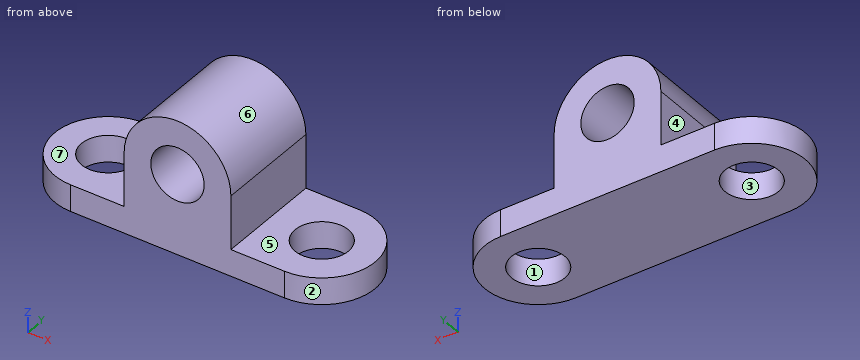
Autodesk Fusion 360 part; units mm, degrees
sketch "Sketch1" plane through (0, 0, 0) normal (0, 0, 1) x (1, 0, 0)
  line L0 (40, -20) -> (-40, -20)
  line L1 (-40, 20) -> (40, 20)
  circle A0 centre (40, 0) radius 10
  circle A1 centre (-40, 0) radius 10
  arc A2 (40, -20) -> (40, 20) centre (40, 0) ccw
  arc A3 (-40, 20) -> (-40, -20) centre (-40, 0) ccw
  dimension "d1" = 80
  dimension "d2" = 40
extrude "Extrude1" add sketch "Sketch1" along normal blind 10
sketch "Sketch2" plane through (0, 0, 0) normal (0, 1, 0) x (1, 0, 0)
  line L0 (-20, -0.1094) -> (20, -0.1094)
  line L1 (20, -0.1094) -> (20, -30.1094)
  line L2 (-20, -30.1094) -> (-20, -0.1094)
  line L3 (-40, 0) -> (-40, -10)
  circle A0 centre (0, -30.1094) radius 20
  circle A1 centre (0, -30.1094) radius 10
  dimension "d9" = 40
  dimension "d10" = 30
  dimension "d11" = 20
  dimension "d12" = 40
  dimension "d13" = 20
extrude "Extrude2" add sketch "Sketch2" along normal mid plane 40
Check sheet for the modelled part. Datum: model origin and axes. Units: mm. Face numbers are marked on the shaded views. A direction names the side the tool comes from. Give positions to 0.01 mm unless a question says otherwise; leave off trailing zeros. Order: outer loops, then holes, each group sorted by start corner. A loop starts at its lowest first (then second) coordinate and runs counter-clockwise, first axis right, second up. Notation, with made-up numbers: M 21.25,6.5 L 55.25,6.5 A17 ccw 55.25,28.5 Z; hole C 37,-18.5 d9. An arc over 180 degrees is marked long. Answer in a Markdown table with one row per item. Add a question column.
Q1. Access from +Z, -Z, +X, -X, +Y, -Y to the whole of each face (thin tool, end or side, straight path). Record for the marked faces 5, 6 and 7.
Q2. Gauge pin test, flat ends, axial feed: pin 1 Ø20 at (x, y) = (42.5, 2.5) entering from +Z; pin 2 Ø10 at (y, z) = (-6, 18.5) entering from +X; pin 3 Ø3 at (y, z) = (13, 12.5) entering from -X; pin 4 Ø12 at (x, z) = (0, 30.11) entering from -Y. Record the tip position at first contact, or that the pin passes through.
Q3. Sectioned sample at B-B, the plane x = 0. Record the boundary of the cut face in (y, z), and give its area (3 significant figures).
Q4. Sectioned sample at A-A, the plane y = 0. Record the boundary of the cut face in (x, z), and give its area (3 significant figures).
Q5. Sectioned sample at C-C, the plane y = 16. Record the boundary of the cut face in (x, z).
Q6. Release check for a two-part mould opening along X. For the marked faces 1, 2, 3 and 4 record: released by +X, released by -X, zero draft, split by the parting line, or undercut.
Q7. Sectioned sample at D-D, the plane z = 35. Record the boundary of the cut face in (x, y), and give its area (3 significant figures).
Q8. Thickness scan on L1, parallel to Y at x = 40, z = 3.25; L2, parallel to X at y = -0.5, z = 30.5; L3, parallel to Z at x = 0, y = -3.5. Record the ranges inside material, lowest first.
Verdict:
| question | item | result |
|---|---|---|
| 1 | face 5 | +Z, +X, +Y, -Y |
| 1 | face 6 | +Z, +Y, -Y |
| 1 | face 7 | +Z, -X, +Y, -Y |
| 2 | pin 1 | z = 10 |
| 2 | pin 2 | x = 20 |
| 2 | pin 3 | x = -20 |
| 2 | pin 4 | through |
| 3 | outline | M -20,0 L 20,0 L 20,20.11 L -20,20.11 Z; M -20,40.11 L 20,40.11 L 20,50.11 L -20,50.11 Z |
| 3 | area | 1,200 mm² |
| 4 | outline | M -60,0 L -50,0 L -50,10 L -60,10 Z; M -30,0 L 30,0 L 30,10 L 20,10 L 20,30.11 A20 ccw -20,30.11 L -20,10 L -30,10 Z; M 50,0 L 60,0 L 60,10 L 50,10 Z; hole C 0,30.11 d20 |
| 4 | area | 1,920 mm² |
| 5 | outline | M -52,0 L 52,0 L 52,10 L 20,10 L 20,30.11 A20 ccw -20,30.11 L -20,10 L -52,10 Z; hole C 0,30.11 d20 |
| 6 | face 1 | undercut |
| 6 | face 2 | released by +X |
| 6 | face 3 | undercut |
| 6 | face 4 | released by -X |
| 7 | outline | M -19.39,-20 L -8.72,-20 L -8.72,20 L -19.39,20 Z; M 8.72,-20 L 19.39,-20 L 19.39,20 L 8.72,20 Z |
| 7 | area | 854 mm² |
| 8 | L1 | -20 to -10, 10 to 20 |
| 8 | L2 | -20 to -9.99, 9.99 to 20 |
| 8 | L3 | 0 to 20.11, 40.11 to 50.11 |
